Input: dimensioned drawing with shaded views. Units: mm. Origin: part minimum x, y, z. A direction names the side the tool comes from. Coordinates: 2 decimals unless noted, no trailing zeros. Order: outer loops, then holes, each group sorted by start corner. A loop starts at its lowest first (then second) coordinate and runs counter-clockwise, first axis right, second up. Notation, with made-up numbers: M -29,17 L -24,17 A22 cw -24,49 Z; hole C 47,66 d9. An arc over 180 degrees is marked long. Write item = value, one per line.
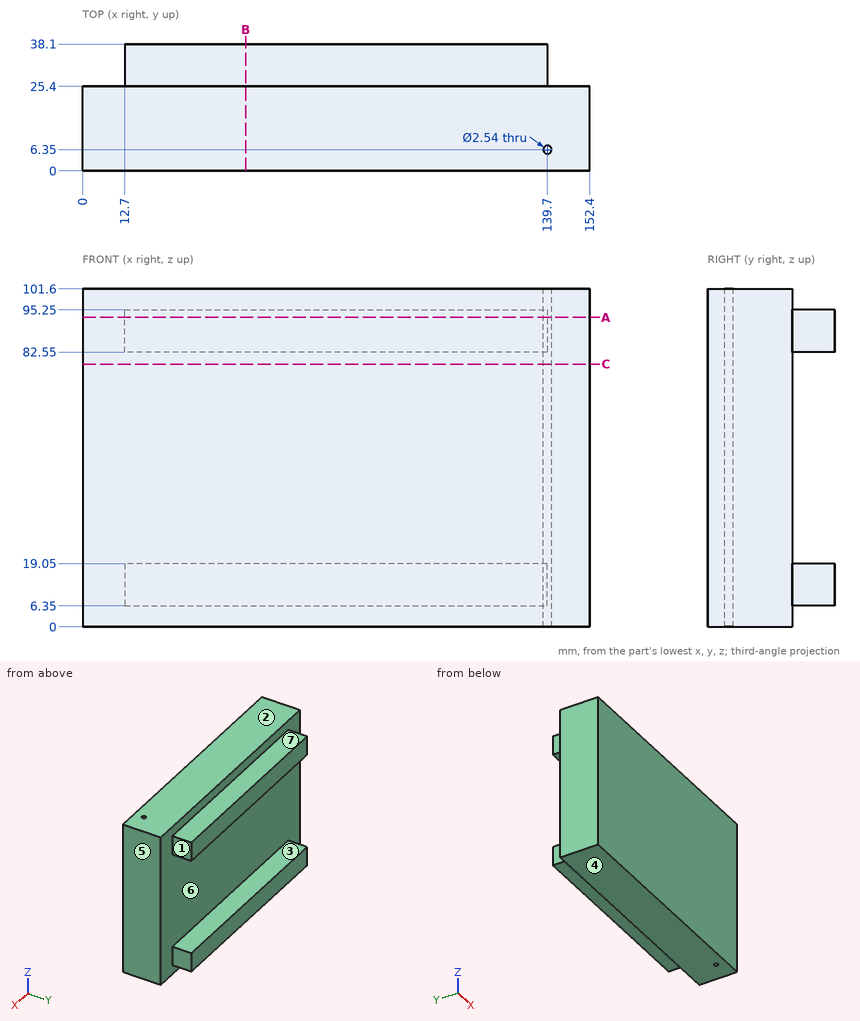
1) Section C-C, the plane z = 79. Return loops of the section in (x, y).
Numbers:
outline = M 0,0 L 152.4,0 L 152.4,25.4 L 0,25.4 Z; hole C 139.7,6.35 d2.54
2) Mould query, pull axis Z, two halves, no side actions, for the marked faces 4, 5, 6 and 7. Classes: pulls with the +Z half, pulls with the -Z half, needs draft (parallel to the pull), parting line crosses it, or undercut.
Numbers:
face_4 = pulls with the -Z half
face_5 = needs draft
face_6 = undercut
face_7 = pulls with the +Z half
3) Pin query (flat end, axial travel): pin 1 (4 mm diameter, centred on x = 49.5, y = 32.5, fed in from +Z); pin 2 (14 mm diameter, centred on x = 56, y = 34.5, fed in from -Z); pin 3 (10 mm diameter, centred on y = 31, z = 12, fed in from -X). Return the tip coordinate at first contact, or that it passes through.
Numbers:
pin_1 = 95.25
pin_2 = 6.35
pin_3 = 12.7
4) Line query: L1, parallel to Z at x = 104.5, y = 27; L2, parallel to X at y = 26.5, z = 86; L3, parallel to Y at x = 68, z = 34.5. Output: solid intervals per line, ascending.
Numbers:
L1 = 6.35 to 19.05, 82.55 to 95.25
L2 = 12.7 to 139.7
L3 = 0 to 25.4
5) Section B-B, the plane x = 49. Return loops of the section in (y, z), and give its area (3 significant figures).
Numbers:
outline = M 0,0 L 25.4,0 L 25.4,6.35 L 38.1,6.35 L 38.1,19.05 L 25.4,19.05 L 25.4,82.55 L 38.1,82.55 L 38.1,95.25 L 25.4,95.25 L 25.4,101.6 L 0,101.6 Z
area = 2,900 mm²
6) Set-up query: the marked faces 1, 2 and 3. Return all of +Z, -Z, +X, -X, +Y, -Y with unobstructed straight access to the full face (end or side cutting, diameter ignored); none if empty.
Numbers:
face_1 = +Z, -Z, +X, +Y
face_2 = +Z, +X, -X, +Y, -Y
face_3 = +X, -X, +Y
7) Section A-A, the plane z = 93. Return loops of the section in (x, y).
Numbers:
outline = M 0,0 L 152.4,0 L 152.4,25.4 L 139.7,25.4 L 139.7,38.1 L 12.7,38.1 L 12.7,25.4 L 0,25.4 Z; hole C 139.7,6.35 d2.54
